```python
from build123d import *

# Parameters (mm, degrees)
SKETCH_1_R               = 46
EXTRUDE_1_DEPTH          = 44
SKETCH_2_R               = 8
EXTRUDE_2_DEPTH          = 44
SKETCH_3_R               = 3.5
CUT_EXTRUDE_1_DEPTH      = 44
PATTERN_CIRCULAR_1_COUNT = 3
EXTRUDE_START            = -52
EXTRUDE_3_DEPTH          = 44
SKETCH_6_R               = 36
CUT_EXTRUDE_2_DEPTH      = 44
HOLE_WIZARD_M10_1_REACH  = 126.34
HOLE_WIZARD_M10_1_BORE_R = 4.25
EXTRUDE_START_2          = 4
EXTRUDE_4_DEPTH          = 9
EXTRUDE_5_DEPTH          = 20
RIB_1_REACH              = 167.714
SKETCH_11_WALL_W         = 368.62723947
SKETCH_11_WALL_H         = 9
EXTRUDE_START_3          = 170
SKETCH_13_W              = 140
SKETCH_13_H              = 64
EXTRUDE_6_DEPTH          = 20
CUT_EXTRUDE_3_DEPTH      = 227.559043166
SKETCH_15_W              = 52
SKETCH_15_H              = 6
CUT_EXTRUDE_4_DEPTH      = 199.557296554
SKETCH_17_W              = 12
SKETCH_17_H              = 20
EXTRUDE_7_DEPTH          = 11


with BuildPart() as part:
    # 草图1 → 凸台-拉伸1 (new body)
    with BuildSketch(Plane(origin=(0, 0, 0), x_dir=(1, 0, 0), z_dir=(0, 1, 0))):
        with Locations(Location((0, 0, 0), (0, 0, 270))):
            Circle(SKETCH_1_R)
    extrude(amount=EXTRUDE_1_DEPTH)

    # 草图2 → 凸台-拉伸2 (add)
    with BuildSketch(Plane(origin=(0, 44, 0), x_dir=(1, 0, 0), z_dir=(0, 1, 0))):
        with Locations((0, -46)):
            Circle(SKETCH_2_R)
    extrude_2 = extrude(amount=-EXTRUDE_2_DEPTH)

    # 草图3 → 切除-拉伸1 (cut)
    with BuildSketch(Plane(origin=(0, 44, 0), x_dir=(1, 0, 0), z_dir=(0, 1, 0))):
        with Locations(Location((0, -46, 0), (0, 0, 270))):
            Circle(SKETCH_3_R)
    cut_extrude_1 = extrude(amount=-CUT_EXTRUDE_1_DEPTH, mode=Mode.SUBTRACT)

    # 阵列(圆周)1: 凸台-拉伸2, 切除-拉伸1 ×3 about axis
    pattern_circular_1_axis = Axis((0, 0, 0), (0, 1, 0))
    add([extrude_2.rotate(pattern_circular_1_axis, i * 360 / PATTERN_CIRCULAR_1_COUNT) for i in range(1, PATTERN_CIRCULAR_1_COUNT)])
    add([cut_extrude_1.rotate(pattern_circular_1_axis, i * 360 / PATTERN_CIRCULAR_1_COUNT) for i in range(1, PATTERN_CIRCULAR_1_COUNT)], mode=Mode.SUBTRACT)

    # 草图5 → 凸台-拉伸3 (add)
    with BuildSketch(Plane.XY.offset(EXTRUDE_START)):
        with BuildLine():
            Line((-12, 27), (-12, 0))
            Line((-12, 0), (12, 0))
            Line((12, 0), (12, 27))
            ThreePointArc((12, 27), (0, 39), (-12, 27))
        make_face()
    extrude(amount=EXTRUDE_3_DEPTH)

    # 草图6 → 切除-拉伸2 (cut)
    with BuildSketch(Plane(origin=(0, 44, 0), x_dir=(1, 0, 0), z_dir=(0, 1, 0))):
        with Locations(Location((0, 0, 0), (0, 0, 270))):
            Circle(SKETCH_6_R)
    extrude(amount=-CUT_EXTRUDE_2_DEPTH, mode=Mode.SUBTRACT)

    # M10 螺纹孔1 bore → M10 螺纹孔1 (cut, up to next)
    with BuildSketch(Plane(origin=(0, 0, -52), x_dir=(-1, 0, 0), z_dir=(0, 0, -1)), mode=Mode.PRIVATE) as hole_wizard_m10_1_sk1:
        with Locations((0, 22)):
            Circle(HOLE_WIZARD_M10_1_BORE_R)
    hole_wizard_m10_1_tool1 = extrude(hole_wizard_m10_1_sk1.sketch, amount=-HOLE_WIZARD_M10_1_REACH, mode=Mode.PRIVATE) & part.part
    add(hole_wizard_m10_1_tool1.solids().sort_by_distance((0, 22, -52))[0], mode=Mode.SUBTRACT)

    # 草图9 → 凸台-拉伸4 (add)
    with BuildSketch(Plane(origin=(0, 0, 0), x_dir=(1, 0, 0), z_dir=(0, 1, 0)).offset(EXTRUDE_START_2)):
        with BuildLine():
            Line((-41, -20.856653615), (-55, -150))
            Line((-55, -150), (55, -150))
            Line((55, -150), (41, -20.856653615))
            ThreePointArc((41, -20.856653615), (27.366589863, -36.973906465), (7.969696861, -45.304347826))
            ThreePointArc((7.969696861, -45.304347826), (0, -54), (-7.969696861, -45.304347826))
            ThreePointArc((-7.969696861, -45.304347826), (-27.366589863, -36.973906465), (-41, -20.856653615))
        make_face()
    extrude(amount=EXTRUDE_4_DEPTH)

    # 草图10 → 凸台-拉伸5 (add)
    with BuildSketch(Plane(origin=(0, 13, 0), x_dir=(1, 0, 0), z_dir=(0, 1, 0))):
        with BuildLine():
            Line((45.947270441, -150), (33.144192236, -31.897688333))
            ThreePointArc((33.144192236, -31.897688333), (37.480880759, -26.668025377), (41, -20.856653615))
            Line((41, -20.856653615), (55, -150))
            Line((55, -150), (45.947270441, -150))
        make_face()
        with BuildLine():
            Line((-33.144192236, -31.897688333), (-45.947270441, -150))
            Line((-45.947270441, -150), (-55, -150))
            Line((-55, -150), (-41, -20.856653615))
            ThreePointArc((-41, -20.856653615), (-37.480880759, -26.668025377), (-33.144192236, -31.897688333))
        make_face()
    extrude(amount=EXTRUDE_5_DEPTH)

    # 草图11 wall → 筋1 (add, up to next)
    with BuildSketch(Plane(origin=(0, 23, 67.516892633), x_dir=(0, -0.568181452229, 0.822903297686), z_dir=(0, -0.822903297686, -0.568181452229)), mode=Mode.PRIVATE) as rib_1_sk1:
        Rectangle(SKETCH_11_WALL_W, SKETCH_11_WALL_H)
    rib_1_tool1 = extrude(rib_1_sk1.sketch, amount=RIB_1_REACH, mode=Mode.PRIVATE) - part.part
    add(rib_1_tool1.solids().sort_by_distance((0, 23, 67.516892633))[0])

    # 草图13 → 凸台-拉伸6 (add)
    with BuildSketch(Plane.XY.offset(EXTRUDE_START_3)):
        with Locations((0, 43)):
            Rectangle(SKETCH_13_W, SKETCH_13_H)
    extrude(amount=-EXTRUDE_6_DEPTH)

    # 草图14 → 切除-拉伸3 (cut, through all)
    with BuildSketch(Plane(origin=(0, 0, 150), x_dir=(-1, 0, 0), z_dir=(0, 0, -1))):
        with BuildLine():
            Line((43, 75), (43, 51))
            ThreePointArc((43, 51), (35, 43), (27, 51))
            Line((27, 51), (27, 75))
            ThreePointArc((27, 75), (35, 83), (43, 75))
        make_face()
    cut_extrude_3 = extrude(amount=-CUT_EXTRUDE_3_DEPTH, mode=Mode.SUBTRACT)

    # 镜向1: 切除-拉伸3 across plane
    add(cut_extrude_3.mirror(Plane(origin=(0, 0, 0), x_dir=(0, 0, 1), z_dir=(1, 0, 0))), mode=Mode.SUBTRACT)

    # 草图15 → 切除-拉伸4 (cut, through all)
    with BuildSketch(Plane(origin=(0, 75, 0), x_dir=(1, 0, 0), z_dir=(0, 1, 0))):
        with Locations((-32, -167)):
            Rectangle(SKETCH_15_W, SKETCH_15_H)
    cut_extrude_4 = extrude(amount=-CUT_EXTRUDE_4_DEPTH, mode=Mode.SUBTRACT)

    # 镜向2: 切除-拉伸4 across plane
    add(cut_extrude_4.mirror(Plane(origin=(0, 0, 0), x_dir=(0, 0, 1), z_dir=(1, 0, 0))), mode=Mode.SUBTRACT)

    # 草图17 → 凸台-拉伸7 (add)
    with BuildSketch(Plane.XZ.offset(-11)):
        with Locations((-64, 160)):
            Rectangle(SKETCH_17_W, SKETCH_17_H)
    extrude_7 = extrude(amount=EXTRUDE_7_DEPTH)

    # 镜向3: 凸台-拉伸7 across plane
    add(extrude_7.mirror(Plane(origin=(0, 0, 0), x_dir=(0, 0, 1), z_dir=(1, 0, 0))))


solid = part.part
```
The listing builds one solid part. Answer for the finished solid, in the listing's coordinates (mm). A direction names the side the tool comes from. Give positions to 0.01 mm unless a question says otherwise; leave off trailing zeros. Write each loop counter-clockwise with the first axis right and the second up, starting at its lowest first coordinate (ties: lowest second). Pieces come first, ordered by that corner, then holes. Notation, with made-up numbers: (-25, 19.5) -> (5, 19.5) arc R26 ccw to (5, 50.5) -> close; hole circle Ø6 at (51, 2.25). An arc over 180 degrees is marked (long way). Use one line per item in the form item = value.
1) For a pull along Z with two mould halves and no side action, classify faces 6 (the flat face through (4.5, 18, 63)), 7 (the flat face through (1, 7, 150)), 8 (the cylindrical face through (5.237, 28.717, 52.048)), 9 (the cylindrical face through (3.37, 19.41, -43.99)) as +Z half, -Z half, draft (parallel to the pull), parting line (faces both ways), or undercut.
Result:
face_6 = undercut
face_7 = +Z half
face_8 = undercut
face_9 = draft
2) Section A-A on z = 0 is taken. Write down the section's boundary in (x, y), plus the area to 3 significant figures.
Result:
outline = (-46, 0) -> (-36, 0) -> (-36, 44) -> (-46, 44) -> close; (36, 0) -> (46, 0) -> (46, 44) -> (36, 44) -> close
area = 880 mm²
3) A tool of negligible diameter and unlimited length cuts with its end or side. For faces 1 (the flat face through (-58, 29.7, 164.3)), 2 (the flat face through (-44, 33, 85)), 3 (the flat face through (-39.456, 22.86, 90.122)), 4 (the flat face through (44, 33, 85)), 5 (the flat face through (-27, 63, 157)), from which of +Z, -Z, +X, -X, +Y, -Y can it reach the whole face along a straight path? Write none if from no direction.
Result:
face_1 = +Z, -Y
face_2 = -X, +Y
face_3 = +Y
face_4 = +X, +Y
face_5 = +Z, -Z, +Y
4) Each of these flat-tipped pins is pushed along its axis until it touches: P1, Ø6.5, axis at x = -41.5, z = 96.5, coming from the +Y side; P2, Ø2, axis at y = 14.5, z = 78.5, coming from the +X side; P3, Ø12, axis at x = 15, y = 18.5, coming from the -Z side; P4, Ø8, axis at y = 51, z = 27.5, coming from the +X side. Where does it stop, or does it pass through?
Result:
P1 = 33
P2 = 47.36
P3 = -52
P4 = through
5) Section C-C on x = -23 is taken. Write down the section's boundary in (y, z).
Result:
outline = (0, -39.84) -> (44, -39.84) -> (44, -27.69) -> (0, -27.69) -> close; (0, 27.69) -> (44, 27.69) -> (44, 39.84) -> (13, 39.84) -> (13, 150) -> (75, 150) -> (75, 164) -> (11, 164) -> (11, 150) -> (4, 150) -> (4, 39.84) -> (0, 39.84) -> close
6) Section B-B on x = 0 is taken. Write down the section's boundary in (y, z), plus the area to 3 significant figures.
Result:
outline = (0, -52) -> (17.75, -52) -> (17.75, -36) -> (0, -36) -> close; (0, 36) -> (44, 36) -> (44, 42.5) -> (0, 42.5) -> close; (0, 49.5) -> (44, 49.5) -> (44, 54) -> (32.33, 54) -> (13, 82) -> (13, 150) -> (75, 150) -> (75, 170) -> (11, 170) -> (11, 150) -> (4, 150) -> (4, 54) -> (0, 54) -> close; (26.25, -52) -> (39, -52) -> (39, -46) -> (44, -46) -> (44, -36) -> (26.25, -36) -> close
area = 3,440 mm²
7) Straight lines are drawn through the part: probe 1 along X at (y, z) = (22, 0); probe 2 along X at (y, z) = (21.5, 46); probe 3 along X at (y, z) = (19, -23). For each, find the intervals that lie inside material, in ascending order.
Result:
probe_1 = -46 to -36, 36 to 46
probe_2 = -43.73 to -34.67, -8 to -3.5, 3.5 to 8, 34.67 to 43.73
probe_3 = -47.84 to -43.34, -36.34 to -27.69, 27.69 to 36.34, 43.34 to 47.84
8) Section D-D on z = 115 is taken. Write down the section's boundary in (x, y).
Result:
outline = (-51.21, 4) -> (51.21, 4) -> (51.21, 33) -> (42.15, 33) -> (42.15, 13) -> (-42.15, 13) -> (-42.15, 33) -> (-51.21, 33) -> close
